```python
from build123d import *

# Parameters (mm, degrees)
F0_R     = 2.413
F1_DEPTH = 12.7
F2_R     = 2.413
F2_R_2   = 36.5125
F3_DEPTH = 3.175
F4_R     = 2.794
F4_R_2   = 38.1
F5_DEPTH = 3.175
F6_R     = 4.953
F6_R_2   = 2.413
F7_DEPTH = 3.175
F8_R     = 4.953
F9_DEPTH = 3.175


with BuildPart() as f1:
    # F0 (on Top) → F1 (new body)
    with BuildSketch(Plane.XY):
        with BuildLine():
            Line((31.75, -41.275), (-31.75, -41.275))
            ThreePointArc((-31.75, -41.275), (-41.275, -50.8), (-31.75, -60.325))
            Line((-31.75, -60.325), (31.75, -60.325))
            Line((31.75, -60.325), (88.9, -60.325))
            Line((88.9, -60.325), (152.4, -60.325))
            ThreePointArc((152.4, -60.325), (161.925, -50.8), (152.4, -41.275))
            Line((152.4, -41.275), (88.9, -41.275))
            ThreePointArc((88.9, -41.275), (82.164808, -38.485192), (79.375, -31.75))
            Line((79.375, -31.75), (79.375, 31.75))
            ThreePointArc((79.375, 31.75), (82.164808, 38.485192), (88.9, 41.275))
            Line((88.9, 41.275), (152.4, 41.275))
            ThreePointArc((152.4, 41.275), (161.925, 50.8), (152.4, 60.325))
            Line((152.4, 60.325), (88.9, 60.325))
            Line((88.9, 60.325), (31.75, 60.325))
            Line((31.75, 60.325), (-31.75, 60.325))
            ThreePointArc((-31.75, 60.325), (-41.275, 50.8), (-31.75, 41.275))
            Line((-31.75, 41.275), (31.75, 41.275))
            ThreePointArc((31.75, 41.275), (38.485192, 38.485192), (41.275, 31.75))
            Line((41.275, 31.75), (41.275, -31.75))
            ThreePointArc((41.275, -31.75), (38.485192, -38.485192), (31.75, -41.275))
        make_face()
        with Locations((-31.75, -50.8)):
            Circle(F0_R, mode=Mode.SUBTRACT)
        with Locations((31.75, -50.8)):
            Circle(F0_R, mode=Mode.SUBTRACT)
        with Locations((88.9, -50.8)):
            Circle(F0_R, mode=Mode.SUBTRACT)
        with Locations((152.4, -50.8)):
            Circle(F0_R, mode=Mode.SUBTRACT)
        with Locations((-31.75, 50.8)):
            Circle(F0_R, mode=Mode.SUBTRACT)
        with Locations((31.75, 50.8)):
            Circle(F0_R, mode=Mode.SUBTRACT)
        with Locations((88.9, 50.8)):
            Circle(F0_R, mode=Mode.SUBTRACT)
        with Locations((152.4, 50.8)):
            Circle(F0_R, mode=Mode.SUBTRACT)
    extrude(amount=F1_DEPTH)

    # F2 (on face) → F3 (join)
    with BuildSketch(Plane(origin=(0, 0, 0), x_dir=(1, 0, 0), z_dir=(0, 0, -1))):
        with BuildLine():
            ThreePointArc((152.4, 41.275), (159.135192, 44.064808), (161.925, 50.8))
            ThreePointArc((161.925, 50.8), (159.135192, 57.535192), (152.4, 60.325))
            Line((152.4, 60.325), (60.325, 60.325))
            Line((60.325, 60.325), (-31.75, 60.325))
            ThreePointArc((-31.75, 60.325), (-38.485192, 57.535192), (-41.275, 50.8))
            ThreePointArc((-41.275, 50.8), (-38.485192, 44.064808), (-31.75, 41.275))
            Line((-31.75, 41.275), (31.75, 41.275))
            ThreePointArc((31.75, 41.275), (38.485192, 38.485192), (41.275, 31.75))
            Line((41.275, 31.75), (41.275, -31.75))
            ThreePointArc((41.275, -31.75), (38.485192, -38.485192), (31.75, -41.275))
            Line((31.75, -41.275), (-31.75, -41.275))
            ThreePointArc((-31.75, -41.275), (-38.485192, -44.064808), (-41.275, -50.8))
            ThreePointArc((-41.275, -50.8), (-38.485192, -57.535192), (-31.75, -60.325))
            Line((-31.75, -60.325), (152.4, -60.325))
            ThreePointArc((152.4, -60.325), (159.135192, -57.535192), (161.925, -50.8))
            ThreePointArc((161.925, -50.8), (159.135192, -44.064808), (152.4, -41.275))
            Line((152.4, -41.275), (88.9, -41.275))
            ThreePointArc((88.9, -41.275), (82.164808, -38.485192), (79.375, -31.75))
            Line((79.375, -31.75), (79.375, 31.75))
            ThreePointArc((79.375, 31.75), (82.164808, 38.485192), (88.9, 41.275))
            Line((88.9, 41.275), (152.4, 41.275))
        make_face()
        with Locations((-31.75, -50.8)):
            Circle(F2_R, mode=Mode.SUBTRACT)
        with Locations((31.75, -50.8)):
            Circle(F2_R, mode=Mode.SUBTRACT)
        with Locations((88.9, -50.8)):
            Circle(F2_R, mode=Mode.SUBTRACT)
        with Locations((152.4, -50.8)):
            Circle(F2_R, mode=Mode.SUBTRACT)
        with Locations((-31.75, 50.8)):
            Circle(F2_R, mode=Mode.SUBTRACT)
        with Locations((31.75, 50.8)):
            Circle(F2_R, mode=Mode.SUBTRACT)
        with Locations((88.9, 50.8)):
            Circle(F2_R, mode=Mode.SUBTRACT)
        with Locations((152.4, 50.8)):
            Circle(F2_R, mode=Mode.SUBTRACT)
        with BuildLine():
            Line((161.925, -50.8), (161.925, 50.8))
            ThreePointArc((161.925, 50.8), (159.135192, 44.064808), (152.4, 41.275))
            Line((152.4, 41.275), (88.9, 41.275))
            ThreePointArc((88.9, 41.275), (82.164808, 38.485192), (79.375, 31.75))
            Line((79.375, 31.75), (79.375, -31.75))
            ThreePointArc((79.375, -31.75), (82.164808, -38.485192), (88.9, -41.275))
            Line((88.9, -41.275), (152.4, -41.275))
            ThreePointArc((152.4, -41.275), (159.135192, -44.064808), (161.925, -50.8))
        make_face()
        with Locations((120.65, 0)):
            Circle(F2_R_2, mode=Mode.SUBTRACT)
        with BuildLine():
            ThreePointArc((-31.75, 41.275), (-38.485192, 44.064808), (-41.275, 50.8))
            Line((-41.275, 50.8), (-41.275, -50.8))
            ThreePointArc((-41.275, -50.8), (-38.485192, -44.064808), (-31.75, -41.275))
            Line((-31.75, -41.275), (31.75, -41.275))
            ThreePointArc((31.75, -41.275), (38.485192, -38.485192), (41.275, -31.75))
            Line((41.275, -31.75), (41.275, 31.75))
            ThreePointArc((41.275, 31.75), (38.485192, 38.485192), (31.75, 41.275))
            Line((31.75, 41.275), (-31.75, 41.275))
        make_face()
        Circle(F2_R_2, mode=Mode.SUBTRACT)
    extrude(amount=F3_DEPTH)

    # F4 (on face) → F5 (join)
    with BuildSketch(Plane(origin=(0, 0, -3.175), x_dir=(1, 0, 0), z_dir=(0, 0, -1))):
        with BuildLine():
            Line((-31.75, -60.325), (152.4, -60.325))
            ThreePointArc((152.4, -60.325), (159.135192, -57.535192), (161.925, -50.8))
            ThreePointArc((161.925, -50.8), (159.135192, -44.064808), (152.4, -41.275))
            Line((152.4, -41.275), (88.9, -41.275))
            ThreePointArc((88.9, -41.275), (82.164808, -38.485192), (79.375, -31.75))
            Line((79.375, -31.75), (79.375, 31.75))
            ThreePointArc((79.375, 31.75), (82.164808, 38.485192), (88.9, 41.275))
            Line((88.9, 41.275), (152.4, 41.275))
            ThreePointArc((152.4, 41.275), (159.135192, 44.064808), (161.925, 50.8))
            ThreePointArc((161.925, 50.8), (159.135192, 57.535192), (152.4, 60.325))
            Line((152.4, 60.325), (-31.75, 60.325))
            ThreePointArc((-31.75, 60.325), (-38.485192, 57.535192), (-41.275, 50.8))
            ThreePointArc((-41.275, 50.8), (-38.485192, 44.064808), (-31.75, 41.275))
            Line((-31.75, 41.275), (31.75, 41.275))
            ThreePointArc((31.75, 41.275), (38.485192, 38.485192), (41.275, 31.75))
            Line((41.275, 31.75), (41.275, -31.75))
            ThreePointArc((41.275, -31.75), (38.485192, -38.485192), (31.75, -41.275))
            Line((31.75, -41.275), (-31.75, -41.275))
            ThreePointArc((-31.75, -41.275), (-38.485192, -44.064808), (-41.275, -50.8))
            ThreePointArc((-41.275, -50.8), (-38.485192, -57.535192), (-31.75, -60.325))
        make_face()
        with Locations((-31.75, -50.8)):
            Circle(F4_R, mode=Mode.SUBTRACT)
        with Locations((31.75, -50.8)):
            Circle(F4_R, mode=Mode.SUBTRACT)
        with Locations((88.9, -50.8)):
            Circle(F4_R, mode=Mode.SUBTRACT)
        with Locations((152.4, -50.8)):
            Circle(F4_R, mode=Mode.SUBTRACT)
        with Locations((-31.75, 50.8)):
            Circle(F4_R, mode=Mode.SUBTRACT)
        with Locations((31.75, 50.8)):
            Circle(F4_R, mode=Mode.SUBTRACT)
        with Locations((88.9, 50.8)):
            Circle(F4_R, mode=Mode.SUBTRACT)
        with Locations((152.4, 50.8)):
            Circle(F4_R, mode=Mode.SUBTRACT)
        with BuildLine():
            Line((-41.275, 50.8), (-41.275, -50.8))
            ThreePointArc((-41.275, -50.8), (-38.485192, -44.064808), (-31.75, -41.275))
            Line((-31.75, -41.275), (31.75, -41.275))
            ThreePointArc((31.75, -41.275), (38.485192, -38.485192), (41.275, -31.75))
            Line((41.275, -31.75), (41.275, 31.75))
            ThreePointArc((41.275, 31.75), (38.485192, 38.485192), (31.75, 41.275))
            Line((31.75, 41.275), (-31.75, 41.275))
            ThreePointArc((-31.75, 41.275), (-38.485192, 44.064808), (-41.275, 50.8))
        make_face()
        Circle(F4_R_2, mode=Mode.SUBTRACT)
        with BuildLine():
            ThreePointArc((152.4, -41.275), (159.135192, -44.064808), (161.925, -50.8))
            Line((161.925, -50.8), (161.925, 50.8))
            ThreePointArc((161.925, 50.8), (159.135192, 44.064808), (152.4, 41.275))
            Line((152.4, 41.275), (88.9, 41.275))
            ThreePointArc((88.9, 41.275), (82.164808, 38.485192), (79.375, 31.75))
            Line((79.375, 31.75), (79.375, -31.75))
            ThreePointArc((79.375, -31.75), (82.164808, -38.485192), (88.9, -41.275))
            Line((88.9, -41.275), (152.4, -41.275))
        make_face()
        with Locations((120.65, 0)):
            Circle(F4_R_2, mode=Mode.SUBTRACT)
    extrude(amount=F5_DEPTH)

    # F6 (on face) → F7 (cut)
    with BuildSketch(Plane.XY.offset(12.7)):
        with Locations((-31.75, 50.8)):
            Circle(F6_R)
        with Locations((-31.75, 50.8)):
            Circle(F6_R_2, mode=Mode.SUBTRACT)
        with Locations((31.75, 50.8)):
            Circle(F6_R)
        with Locations((31.75, 50.8)):
            Circle(F6_R_2, mode=Mode.SUBTRACT)
        with Locations((88.9, 50.8)):
            Circle(F6_R)
        with Locations((88.9, 50.8)):
            Circle(F6_R_2, mode=Mode.SUBTRACT)
        with Locations((152.4, 50.8)):
            Circle(F6_R)
        with Locations((152.4, 50.8)):
            Circle(F6_R_2, mode=Mode.SUBTRACT)
        with Locations((-31.75, -50.8)):
            Circle(F6_R)
        with Locations((-31.75, -50.8)):
            Circle(F6_R_2, mode=Mode.SUBTRACT)
        with Locations((31.75, -50.8)):
            Circle(F6_R)
        with Locations((31.75, -50.8)):
            Circle(F6_R_2, mode=Mode.SUBTRACT)
        with Locations((88.9, -50.8)):
            Circle(F6_R)
        with Locations((88.9, -50.8)):
            Circle(F6_R_2, mode=Mode.SUBTRACT)
        with Locations((152.4, -50.8)):
            Circle(F6_R)
        with Locations((152.4, -50.8)):
            Circle(F6_R_2, mode=Mode.SUBTRACT)
    extrude(amount=-F7_DEPTH, mode=Mode.SUBTRACT)

    # F8 (on face) → F9 (cut)
    with BuildSketch(Plane(origin=(0, 0, -6.35), x_dir=(1, 0, 0), z_dir=(0, 0, -1))):
        with Locations((-31.75, 50.8)):
            Circle(F8_R)
        with Locations((31.75, 50.8)):
            Circle(F8_R)
        with Locations((88.9, 50.8)):
            Circle(F8_R)
        with Locations((152.4, 50.8)):
            Circle(F8_R)
        with Locations((-31.75, -50.8)):
            Circle(F8_R)
        with Locations((31.75, -50.8)):
            Circle(F8_R)
        with Locations((88.9, -50.8)):
            Circle(F8_R)
        with Locations((152.4, -50.8)):
            Circle(F8_R)
    extrude(amount=-F9_DEPTH, mode=Mode.SUBTRACT)


solid = f1.part
```
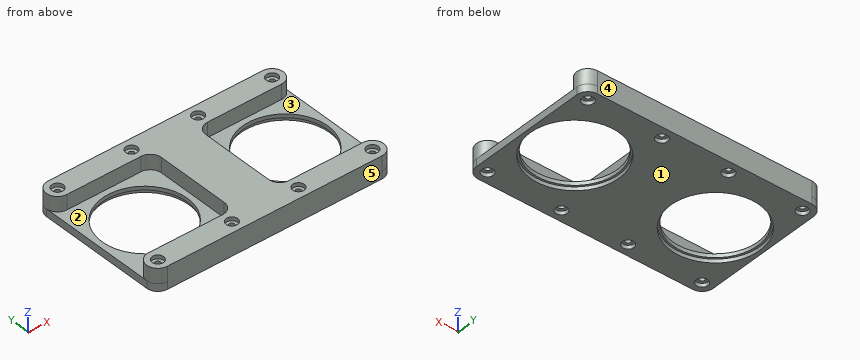
Design review of the part built by this model. Coordinates are the model's own, in mm. Face numbers are marked on the shaded views. A direction names the side the tool comes from. Coordinates: 2 decimals unless noted, no trailing zeros. Write each loop counter-clockwise with the first axis right and the second up, starting at its lowest first coordinate (ties: lowest second). Pieces come first, ordered by that corner, then holes.
1) Add section A-A (y = 0). State how many separate pieces and enclosed holes the cut face has, plus the area to 3 significant figures.
2) Add section D-D (x = 20.5). Write out the cut boundary in (y, z) (3 decimals).
3) To check wall thickness, follow L1, parallel to X at y = 0, z = -1.9 (1 decimal); L2, parallel to Y at x = 88.9, z = 12.15 (3 decimals); L3, parallel to Y at x = 152.4, z = 6.75 (3 decimals). State the ranges of each line that lie inside material, in increasing order.
4) Machinability: for the marked faces 1 and 2, which of the approach directions +Z, -Z, +X, -X, +Y, -Y give a long, thin tool a straight path to every point of the face, cutting with its end or side? Answer none if there is none.
5) Mouldability with a two-part tool opening along Y and no side actions: class the marked faces 3, 4 and 5 as +Y half, -Y half, draft (parallel to the pull), parting line (faces both ways), or undercut.
6) Insertion check: pin 1 (6 mm diameter, centred on x = 152.4, y = 50.8, fed in from +Z) (3 decimals); pin 2 (3 mm diameter, centred on x = -34, y = 52.5, fed in from -Z) (3 decimals); pin 3 (5 mm diameter, centred on x = 87, y = 53, fed in from -Z); pin 4 (4 mm diameter, centred on x = 88.9, y = 50.8, fed in from -Z). Each pin has a flat end and moves straight along its axis. Give the tip position at first contact, or say it passes through.
Check result:
1. separate pieces: 3
1. enclosed holes: 0
1. area: 827 mm2
2. outline: (-60.325, -6.35) - (-32.115, -6.35) - (-32.115, -3.175) - (-30.214, -3.175) - (-30.214, 0) - (-41.275, 0) - (-41.275, 12.7) - (-60.325, 12.7) - close; (30.214, -3.175) - (32.115, -3.175) - (32.115, -6.35) - (60.325, -6.35) - (60.325, 12.7) - (41.275, 12.7) - (41.275, 0) - (30.214, 0) - close
3. L1: x = -41.3 to -36.5, 36.5 to 84.1, 157.2 to 161.9
3. L2: y = -60.325 to -55.753, -45.847 to -41.275, 41.275 to 45.847, 55.753 to 60.325
3. L3: y = -60.325 to -53.213, -48.387 to -41.275, 41.275 to 48.387, 53.213 to 60.325
4. face 1: -Z, +X, -X, +Y, -Y
4. face 2: +Z, -X
5. face 3: undercut
5. face 4: +Y half
5. face 5: -Y half
6. pin 1: stops at z = 9.525
6. pin 2: stops at z = -3.175
6. pin 3: stops at z = -6.35
6. pin 4: passes through
